```python
from build123d import *

# Parameters (mm, degrees)
ESBO_O1_W                = 231.5
ESBO_O1_H                = 170
ESBO_O1_R                = 4
RESSALTO_EXTRUS_O1_DEPTH = 6
ESBO_O6_W                = 17.807692308
ESBO_O6_H                = 6
ESBO_O6_W_2              = 17.78
CORTE_EXTRUS_O1_DEPTH    = 6
CORTE_EXTRUS_O2_REACH    = 145.733
ESBO_O7_W                = 6
ESBO_O7_H                = 15.454545455


with BuildPart() as part:
    # Esboço1 → Ressalto-extrusão1 (new body)
    with BuildSketch(Plane(origin=(0, 0, 0), x_dir=(1, 0, 0), z_dir=(0, 1, 0))):
        Rectangle(ESBO_O1_W, ESBO_O1_H)
        with Locations(Location((-81, 54, 0), (0, 0, 270))):
            Circle(ESBO_O1_R, mode=Mode.SUBTRACT)
        with Locations(Location((-54, 54, 0), (0, 0, 270))):
            Circle(ESBO_O1_R, mode=Mode.SUBTRACT)
        with Locations(Location((-27, 54, 0), (0, 0, 270))):
            Circle(ESBO_O1_R, mode=Mode.SUBTRACT)
        with Locations(Location((0, 54, 0), (0, 0, 270))):
            Circle(ESBO_O1_R, mode=Mode.SUBTRACT)
        with Locations(Location((27, 54, 0), (0, 0, 270))):
            Circle(ESBO_O1_R, mode=Mode.SUBTRACT)
        with Locations(Location((54, 54, 0), (0, 0, 270))):
            Circle(ESBO_O1_R, mode=Mode.SUBTRACT)
        with Locations(Location((81, 54, 0), (0, 0, 270))):
            Circle(ESBO_O1_R, mode=Mode.SUBTRACT)
        with Locations(Location((-54, 27, 0), (0, 0, 270))):
            Circle(ESBO_O1_R, mode=Mode.SUBTRACT)
        with Locations(Location((-27, 27, 0), (0, 0, 270))):
            Circle(ESBO_O1_R, mode=Mode.SUBTRACT)
        with Locations(Location((0, 27, 0), (0, 0, 270))):
            Circle(ESBO_O1_R, mode=Mode.SUBTRACT)
        with Locations(Location((27, 27, 0), (0, 0, 270))):
            Circle(ESBO_O1_R, mode=Mode.SUBTRACT)
        with Locations(Location((54, 27, 0), (0, 0, 270))):
            Circle(ESBO_O1_R, mode=Mode.SUBTRACT)
        with Locations(Location((81, 27, 0), (0, 0, 270))):
            Circle(ESBO_O1_R, mode=Mode.SUBTRACT)
        with Locations(Location((-54, 0, 0), (0, 0, 270))):
            Circle(ESBO_O1_R, mode=Mode.SUBTRACT)
        with Locations(Location((-27, 0, 0), (0, 0, 270))):
            Circle(ESBO_O1_R, mode=Mode.SUBTRACT)
        with Locations(Location((0, 0, 0), (0, 0, 270))):
            Circle(ESBO_O1_R, mode=Mode.SUBTRACT)
        with Locations(Location((27, 0, 0), (0, 0, 270))):
            Circle(ESBO_O1_R, mode=Mode.SUBTRACT)
        with Locations(Location((54, 0, 0), (0, 0, 270))):
            Circle(ESBO_O1_R, mode=Mode.SUBTRACT)
        with Locations(Location((81, 0, 0), (0, 0, 270))):
            Circle(ESBO_O1_R, mode=Mode.SUBTRACT)
        with Locations(Location((-54, -27, 0), (0, 0, 270))):
            Circle(ESBO_O1_R, mode=Mode.SUBTRACT)
        with Locations(Location((-27, -27, 0), (0, 0, 270))):
            Circle(ESBO_O1_R, mode=Mode.SUBTRACT)
        with Locations(Location((0, -27, 0), (0, 0, 270))):
            Circle(ESBO_O1_R, mode=Mode.SUBTRACT)
        with Locations(Location((27, -27, 0), (0, 0, 270))):
            Circle(ESBO_O1_R, mode=Mode.SUBTRACT)
        with Locations(Location((54, -27, 0), (0, 0, 270))):
            Circle(ESBO_O1_R, mode=Mode.SUBTRACT)
        with Locations(Location((81, -27, 0), (0, 0, 270))):
            Circle(ESBO_O1_R, mode=Mode.SUBTRACT)
        with Locations(Location((-54, -54, 0), (0, 0, 270))):
            Circle(ESBO_O1_R, mode=Mode.SUBTRACT)
        with Locations(Location((-27, -54, 0), (0, 0, 270))):
            Circle(ESBO_O1_R, mode=Mode.SUBTRACT)
        with Locations(Location((0, -54, 0), (0, 0, 270))):
            Circle(ESBO_O1_R, mode=Mode.SUBTRACT)
        with Locations(Location((27, -54, 0), (0, 0, 270))):
            Circle(ESBO_O1_R, mode=Mode.SUBTRACT)
        with Locations(Location((54, -54, 0), (0, 0, 270))):
            Circle(ESBO_O1_R, mode=Mode.SUBTRACT)
        with Locations(Location((81, -54, 0), (0, 0, 270))):
            Circle(ESBO_O1_R, mode=Mode.SUBTRACT)
        with Locations(Location((-81, 27, 0), (0, 0, 270))):
            Circle(ESBO_O1_R, mode=Mode.SUBTRACT)
        with Locations(Location((-81, 0, 0), (0, 0, 270))):
            Circle(ESBO_O1_R, mode=Mode.SUBTRACT)
        with Locations(Location((-81, -27, 0), (0, 0, 270))):
            Circle(ESBO_O1_R, mode=Mode.SUBTRACT)
        with Locations(Location((-81, -54, 0), (0, 0, 270))):
            Circle(ESBO_O1_R, mode=Mode.SUBTRACT)
    extrude(amount=RESSALTO_EXTRUS_O1_DEPTH)

    # Esboço6 → Corte-extrusão1 (cut)
    with BuildSketch(Plane.XZ):
        with Locations((-106.846153846, 82)):
            Rectangle(ESBO_O6_W, ESBO_O6_H)
        with Locations((-71.226153846, 82)):
            Rectangle(ESBO_O6_W, ESBO_O6_H)
        with Locations((-35.606153846, 82)):
            Rectangle(ESBO_O6_W, ESBO_O6_H)
        with Locations((0.013846154, 82)):
            Rectangle(ESBO_O6_W, ESBO_O6_H)
        with Locations((35.633846154, 82)):
            Rectangle(ESBO_O6_W, ESBO_O6_H)
        with Locations((71.253846154, 82)):
            Rectangle(ESBO_O6_W, ESBO_O6_H)
        with Locations((106.86, 82)):
            Rectangle(ESBO_O6_W_2, ESBO_O6_H)
        with Locations((106.86, -82)):
            Rectangle(ESBO_O6_W_2, ESBO_O6_H)
        with Locations((71.253846154, -82)):
            Rectangle(ESBO_O6_W, ESBO_O6_H)
        with Locations((35.633846154, -82)):
            Rectangle(ESBO_O6_W, ESBO_O6_H)
        with Locations((0.013846154, -82)):
            Rectangle(ESBO_O6_W, ESBO_O6_H)
        with Locations((-35.606153846, -82)):
            Rectangle(ESBO_O6_W, ESBO_O6_H)
        with Locations((-71.226153846, -82)):
            Rectangle(ESBO_O6_W, ESBO_O6_H)
        with Locations((-106.846153846, -82)):
            Rectangle(ESBO_O6_W, ESBO_O6_H)
    extrude(amount=-CORTE_EXTRUS_O1_DEPTH, mode=Mode.SUBTRACT)

    # Esboço7 → Corte-extrusão2 (cut, up to next)
    with BuildSketch(Plane.XZ, mode=Mode.PRIVATE) as corte_extrus_o2_sk1:
        with Locations((112.75, -77.272727272)):
            Rectangle(ESBO_O7_W, ESBO_O7_H)
    corte_extrus_o2_tool1 = extrude(corte_extrus_o2_sk1.sketch, amount=-CORTE_EXTRUS_O2_REACH, mode=Mode.PRIVATE) & part.part
    # Esboço7 → Corte-extrusão2 (cut, up to next)
    with BuildSketch(Plane.XZ, mode=Mode.PRIVATE) as corte_extrus_o2_sk2:
        with Locations((-112.75, -77.272727272)):
            Rectangle(ESBO_O7_W, ESBO_O7_H)
    corte_extrus_o2_tool2 = extrude(corte_extrus_o2_sk2.sketch, amount=-CORTE_EXTRUS_O2_REACH, mode=Mode.PRIVATE) & part.part
    # Esboço7 → Corte-extrusão2 (cut, up to next)
    with BuildSketch(Plane.XZ, mode=Mode.PRIVATE) as corte_extrus_o2_sk3:
        with Locations((112.75, -46.362727273)):
            Rectangle(ESBO_O7_W, ESBO_O7_H)
    corte_extrus_o2_tool3 = extrude(corte_extrus_o2_sk3.sketch, amount=-CORTE_EXTRUS_O2_REACH, mode=Mode.PRIVATE) & part.part
    # Esboço7 → Corte-extrusão2 (cut, up to next)
    with BuildSketch(Plane.XZ, mode=Mode.PRIVATE) as corte_extrus_o2_sk4:
        with Locations((112.75, -15.452727273)):
            Rectangle(ESBO_O7_W, ESBO_O7_H)
    corte_extrus_o2_tool4 = extrude(corte_extrus_o2_sk4.sketch, amount=-CORTE_EXTRUS_O2_REACH, mode=Mode.PRIVATE) & part.part
    # Esboço7 → Corte-extrusão2 (cut, up to next)
    with BuildSketch(Plane.XZ, mode=Mode.PRIVATE) as corte_extrus_o2_sk5:
        with Locations((112.75, 15.457272728)):
            Rectangle(ESBO_O7_W, ESBO_O7_H)
    corte_extrus_o2_tool5 = extrude(corte_extrus_o2_sk5.sketch, amount=-CORTE_EXTRUS_O2_REACH, mode=Mode.PRIVATE) & part.part
    # Esboço7 → Corte-extrusão2 (cut, up to next)
    with BuildSketch(Plane.XZ, mode=Mode.PRIVATE) as corte_extrus_o2_sk6:
        with Locations((112.75, 46.367272728)):
            Rectangle(ESBO_O7_W, ESBO_O7_H)
    corte_extrus_o2_tool6 = extrude(corte_extrus_o2_sk6.sketch, amount=-CORTE_EXTRUS_O2_REACH, mode=Mode.PRIVATE) & part.part
    # Esboço7 → Corte-extrusão2 (cut, up to next)
    with BuildSketch(Plane.XZ, mode=Mode.PRIVATE) as corte_extrus_o2_sk7:
        with Locations((112.75, 77.277272728)):
            Rectangle(ESBO_O7_W, ESBO_O7_H)
    corte_extrus_o2_tool7 = extrude(corte_extrus_o2_sk7.sketch, amount=-CORTE_EXTRUS_O2_REACH, mode=Mode.PRIVATE) & part.part
    # Esboço7 → Corte-extrusão2 (cut, up to next)
    with BuildSketch(Plane.XZ, mode=Mode.PRIVATE) as corte_extrus_o2_sk8:
        with Locations((-112.75, -46.362727273)):
            Rectangle(ESBO_O7_W, ESBO_O7_H)
    corte_extrus_o2_tool8 = extrude(corte_extrus_o2_sk8.sketch, amount=-CORTE_EXTRUS_O2_REACH, mode=Mode.PRIVATE) & part.part
    # Esboço7 → Corte-extrusão2 (cut, up to next)
    with BuildSketch(Plane.XZ, mode=Mode.PRIVATE) as corte_extrus_o2_sk9:
        with Locations((-112.75, -15.452727273)):
            Rectangle(ESBO_O7_W, ESBO_O7_H)
    corte_extrus_o2_tool9 = extrude(corte_extrus_o2_sk9.sketch, amount=-CORTE_EXTRUS_O2_REACH, mode=Mode.PRIVATE) & part.part
    # Esboço7 → Corte-extrusão2 (cut, up to next)
    with BuildSketch(Plane.XZ, mode=Mode.PRIVATE) as corte_extrus_o2_sk10:
        with Locations((-112.75, 15.457272728)):
            Rectangle(ESBO_O7_W, ESBO_O7_H)
    corte_extrus_o2_tool10 = extrude(corte_extrus_o2_sk10.sketch, amount=-CORTE_EXTRUS_O2_REACH, mode=Mode.PRIVATE) & part.part
    # Esboço7 → Corte-extrusão2 (cut, up to next)
    with BuildSketch(Plane.XZ, mode=Mode.PRIVATE) as corte_extrus_o2_sk11:
        with Locations((-112.75, 46.367272728)):
            Rectangle(ESBO_O7_W, ESBO_O7_H)
    corte_extrus_o2_tool11 = extrude(corte_extrus_o2_sk11.sketch, amount=-CORTE_EXTRUS_O2_REACH, mode=Mode.PRIVATE) & part.part
    # Esboço7 → Corte-extrusão2 (cut, up to next)
    with BuildSketch(Plane.XZ, mode=Mode.PRIVATE) as corte_extrus_o2_sk12:
        with Locations((-112.75, 77.277272728)):
            Rectangle(ESBO_O7_W, ESBO_O7_H)
    corte_extrus_o2_tool12 = extrude(corte_extrus_o2_sk12.sketch, amount=-CORTE_EXTRUS_O2_REACH, mode=Mode.PRIVATE) & part.part
    add(corte_extrus_o2_tool1.solids().sort_by_distance((112.75, 0, -77.272727))[0], mode=Mode.SUBTRACT)
    add(corte_extrus_o2_tool2.solids().sort_by_distance((-112.75, 0, -77.272727))[0], mode=Mode.SUBTRACT)
    add(corte_extrus_o2_tool3.solids().sort_by_distance((112.75, 0, -46.362727))[0], mode=Mode.SUBTRACT)
    add(corte_extrus_o2_tool4.solids().sort_by_distance((112.75, 0, -15.452727))[0], mode=Mode.SUBTRACT)
    add(corte_extrus_o2_tool5.solids().sort_by_distance((112.75, 0, 15.457273))[0], mode=Mode.SUBTRACT)
    add(corte_extrus_o2_tool6.solids().sort_by_distance((112.75, 0, 46.367273))[0], mode=Mode.SUBTRACT)
    add(corte_extrus_o2_tool7.solids().sort_by_distance((112.75, 0, 77.277273))[0], mode=Mode.SUBTRACT)
    add(corte_extrus_o2_tool8.solids().sort_by_distance((-112.75, 0, -46.362727))[0], mode=Mode.SUBTRACT)
    add(corte_extrus_o2_tool9.solids().sort_by_distance((-112.75, 0, -15.452727))[0], mode=Mode.SUBTRACT)
    add(corte_extrus_o2_tool10.solids().sort_by_distance((-112.75, 0, 15.457273))[0], mode=Mode.SUBTRACT)
    add(corte_extrus_o2_tool11.solids().sort_by_distance((-112.75, 0, 46.367273))[0], mode=Mode.SUBTRACT)
    add(corte_extrus_o2_tool12.solids().sort_by_distance((-112.75, 0, 77.277273))[0], mode=Mode.SUBTRACT)


solid = part.part
```
Check sheet for the modelled part. Datum: model origin and axes. Units: mm. A direction names the side the tool comes from. Round coordinates to 2 decimals unless told otherwise and drop trailing zeros. Order: outer loops, then holes, each group sorted by start corner. A loop starts at its lowest first (then second) coordinate and runs counter-clockwise, first axis right, second up. Notation, with made-up numbers: (6.5, 46) - (45.5, 46) arc R10 ccw to (45.5, 62) - close; hole circle Ø5 at (-17, 88.5). An arc over 180 degrees is marked (long way). Answer as CSV lines item,"result". Start each with the question number.
1) Tool access check on faces 4 (the face through (-113, 3, 23.185)), 5 (the face through (-71, 3, -79)), 6 (the face through (113, 3, -69.545)), 7 (the face through (113, 3, 69.55)). Record the directions out of +Z, -Z, +X, -X, +Y, -Y that give a thin tool (end or side, any length) a straight path to the whole face; none if there is none.
2) Section check B-B (z = -27). Give the number of separate pieces and of enclosed holes in the cut face, then the cut area to 3 significant figures.
3) Depth check by flat-ended pin: pin 1 (1.8 mm diameter, centred on y = 4.5, z = -83.5, fed in from +X); pin 2 (1.8 mm diameter, centred on x = -103.5, y = 2, fed in from -Z); pin 3 (1.8 mm diameter, centred on y = 2, z = 42.5, fed in from -X). Enter the tip coordinate at first touch or a pass-through.
4) Section check D-D (x = 54). Record the cut outline in (y, z), then the cut area to 3 significant figures.
5) Section check A-A (x = 0). Record the cut outline in (y, z).
6) Scan lines: probe 1 along Z at (x, y) = (56, 1.95); probe 2 along X at (y, z) = (3.8, 70); probe 3 along Z at (x, y) = (-70.5, 4.1). Record each from-to range of solid material in increasing order.
7) Draft check along Z on faces 1 (the face through (50.451, 2.958, -52.154)), 2 (the face through (-44.51, 3, 82)), 3 (the face through (36, 3, 79)). Enter one of: +Z half, -Z half, draft (parallel to the pull), parting line (faces both ways), or undercut.
Determined:
1,face 4,"-X, +Y, -Y"
1,face 5,"-Z, +Y, -Y"
1,face 6,"-Z, +X, +Y, -Y"
1,face 7,"+Z, +X, +Y, -Y"
2,separate pieces,"8"
2,enclosed holes,"0"
2,area,"1,050 mm^2"
3,pin 1,"x = 97.97"
3,pin 2,"z = -79"
3,pin 3,"x = -109.75"
4,outline,"(0, -85) - (6, -85) - (6, -58) - (0, -58) - close; (0, -50) - (6, -50) - (6, -31) - (0, -31) - close; (0, -23) - (6, -23) - (6, -4) - (0, -4) - close; (0, 4) - (6, 4) - (6, 23) - (0, 23) - close; (0, 31) - (6, 31) - (6, 50) - (0, 50) - close; (0, 58) - (6, 58) - (6, 85) - (0, 85) - close"
4,area,"780 mm^2"
5,outline,"(0, -79) - (6, -79) - (6, -58) - (0, -58) - close; (0, -50) - (6, -50) - (6, -31) - (0, -31) - close; (0, -23) - (6, -23) - (6, -4) - (0, -4) - close; (0, 4) - (6, 4) - (6, 23) - (0, 23) - close; (0, 31) - (6, 31) - (6, 50) - (0, 50) - close; (0, 58) - (6, 58) - (6, 79) - (0, 79) - close"
6,probe 1,"-85 to -57.46, -50.54 to -30.46, -23.54 to -3.46, 3.46 to 23.54, 30.46 to 50.54, 57.46 to 85"
6,probe 2,"-109.75 to 109.75"
6,probe 3,"-79 to 79"
7,face 1,"undercut"
7,face 2,"draft"
7,face 3,"+Z half"
